Read the model definition and answer for the solid it produces. Units are mm, in the model's axes. A direction names the side the tool comes from. Coordinates: 2 decimals unless noted, no trailing zeros. Order: outer loops, then holes, each group sorted by start corner. A loop starts at its lowest first (then second) coordinate and runs counter-clockwise, first axis right, second up. Notation, with made-up numbers: (3, 2) -> (12, 2) arc R32 ccw to (12, 36) -> close; hole circle Ø11 at (32.25, 29). An arc over 180 degrees is marked (long way). Use CSV: the item, a comma, the result in double quotes.
```python
from build123d import *

# Parameters (mm, degrees)
SKETCH005_R         = 2
EXTRUDE002_DEPTH    = 20
SKETCH002_R         = 7.75
EXTRUDE_DEPTH       = 16
BOX_W               = 8
BOX_H               = 74
BOX_DEPTH           = 120
PAD001_DEPTH        = 20
PAD_DEPTH           = 20
HOLE_D              = 4.4
HOLE_CBORE_D        = 8
HOLE_CBORE_DEPTH    = 2.4
HOLE001_D           = 1.75
HOLE001_CBORE_D     = 3.2
HOLE001_CBORE_DEPTH = 0.96
BOX001_W            = 65
BOX001_H            = 8
BOX001_DEPTH        = 120
BOX002_W            = 2
BOX002_H            = 10
BOX002_DEPTH        = 10
EXTRUDE001_DEPTH    = 8
CHAMFER_SIZE        = 2.5


with BuildPart() as extrude002:
    # Sketch005 (on Face21 of Fusion001) → Extrude002 (new body)
    with BuildSketch(Plane(origin=(-8, 0, 0), x_dir=(0, -1, 0), z_dir=(-1, 0, 0))):
        with Locations((-55, 60)):
            Circle(SKETCH005_R)
        with Locations((-22, 60)):
            Circle(SKETCH005_R)
    extrude(amount=EXTRUDE002_DEPTH)


with BuildPart() as extrude002_1:
    # Extrude002 placement: moved
    add(extrude002.part.moved(Location((16, 0, 0))))


with BuildPart() as extrude_body:
    # Sketch002 (on Face9 of Fusion) → Extrude (new body)
    with BuildSketch(Plane(origin=(0, 74, 0), x_dir=(-1, 0, 0), z_dir=(0, 1, 0))):
        with Locations((35, 60)):
            Circle(SKETCH002_R)
    extrude(amount=EXTRUDE_DEPTH)


with BuildPart() as cube:
    # Box → Box (new body)
    with BuildSketch(Plane(origin=(-8, 0, 0), x_dir=(1, 0, 0), z_dir=(0, 0, 1))):
        with Locations((4, 37)):
            Rectangle(BOX_W, BOX_H)
    extrude(amount=BOX_DEPTH)


with BuildPart() as body001:
    # Sketch001 → Pad001 (new body)
    with BuildSketch(Plane.XY):
        Polygon((-88, 8), (-8, 8), (-8, 36), (-78, 36), (-78, 44), (-8, 44), (-8, 66), (-65, 66), (-65, 74), (0, 74), (0, 0), (-88, 0), align=None)
    extrude(amount=PAD001_DEPTH)


with BuildPart() as body001_1:
    # Body001 placement: moved
    add(body001.part.moved(Location((0, 0, 100))))


with BuildPart() as body:
    # Sketch → Pad (new body)
    with BuildSketch(Plane.XY):
        Polygon((-88, 8), (-8, 8), (-8, 36), (-78, 36), (-78, 44), (-8, 44), (-8, 66), (-65, 66), (-65, 74), (0, 74), (0, 0), (-88, 0), align=None)
    extrude(amount=PAD_DEPTH)

    # Hole (through all)
    with Locations(Plane(origin=(-8, 0, 0), x_dir=(0, -1, 0), z_dir=(-1, 0, 0))):
        with Locations((-55, 60), (-22, 60)):
            CounterBoreHole(HOLE_D / 2, HOLE_CBORE_D / 2, HOLE_CBORE_DEPTH)

    # Hole001 (through all)
    with Locations(Plane(origin=(-8, 0, 0), x_dir=(0, -1, 0), z_dir=(-1, 0, 0))):
        with Locations((-55, 60), (-22, 60)):
            CounterBoreHole(HOLE001_D / 2, HOLE001_CBORE_D / 2, HOLE001_CBORE_DEPTH)


with BuildPart() as fusion:
    # Box001 → Box001 (new body)
    with BuildSketch(Plane(origin=(-65, 66, 0), x_dir=(1, 0, 0), z_dir=(0, 0, 1))):
        with Locations((32.5, 4)):
            Rectangle(BOX001_W, BOX001_H)
    extrude(amount=BOX001_DEPTH)

    # Fusion: union Cube, Body001, Body
    add(cube.part)
    add(body001_1.part)
    add(body.part)


with BuildPart() as cube002:
    # Box002 → Box002 (new body)
    with BuildSketch(Plane(origin=(-84, 64, 55), x_dir=(1, 0, 0), z_dir=(0, 0, 1))):
        with Locations((1, 5)):
            Rectangle(BOX002_W, BOX002_H)
    extrude(amount=BOX002_DEPTH)


with BuildPart() as chamfer_body:
    # Sketch003 (on Face9 of Fusion) → Extrude001 (new body)
    with BuildSketch(Plane(origin=(0, 74, 0), x_dir=(-1, 0, 0), z_dir=(0, 1, 0))):
        Polygon((65, 100), (65, 20), (88, 50), (88, 70), align=None)
    extrude(amount=-EXTRUDE001_DEPTH)

    # Cut: cut Cube002
    add(cube002.part, mode=Mode.SUBTRACT)

    # Fusion001: union Extrude body, Fusion
    add(extrude_body.part)
    add(fusion.part)

    # Cut001: cut Extrude002
    add(extrude002_1.part, mode=Mode.SUBTRACT)

    # Chamfer
    chamfer_edges = [chamfer_body.edges().sort_by_distance(p)[0] for p in [
        (-8, 24, 60),
        (-8, 57, 60),
    ]]
    chamfer(chamfer_edges, length=CHAMFER_SIZE)


solid = chamfer_body.part
```
Item 1: The mould has two halves that part along Y. Classify faces 1 (the flat face through (-34, 0, 19)), 2 (the cylindrical face through (-3, 55, 62)), 3 (the flat face through (-65, 70, 10)): +Y half, -Y half, draft (parallel to the pull), parting line (faces both ways), or undercut.
Return value:
face 1,"-Y half"
face 2,"undercut"
face 3,"draft"
Item 2: Straight lines are drawn through the part: line 1 along Y through (x, z) = (-3.45, 60); line 2 along Y through (x, z) = (-54, 103); line 3 along Z through (x, y) = (-1.2, 22). For each, find the intervals that lie inside material, in ascending order.
Return value:
line 1,"y = 0 to 20, 24 to 53, 57 to 74"
line 2,"y = 0 to 8, 36 to 44, 66 to 74"
line 3,"z = 0 to 58, 62 to 120"
Item 3: Find section D-D, the plane x = -16. Give the vertices of the cut face in (y, z).
Return value:
outline,"(0, 0) -> (8, 0) -> (8, 20) -> (0, 20) -> close; (0, 100) -> (8, 100) -> (8, 120) -> (0, 120) -> close; (36, 0) -> (44, 0) -> (44, 20) -> (36, 20) -> close; (36, 100) -> (44, 100) -> (44, 120) -> (36, 120) -> close; (66, 0) -> (74, 0) -> (74, 120) -> (66, 120) -> close"
Item 4: Each of these flat-tipped pins is pushed along its axis until it touches: P1, Ø4, axis at y = 69.5, z = 113.5, coming from the -X side; P2, Ø8, axis at y = 49.5, z = 61.5, coming from the +X side; P3, Ø9, axis at y = 40, z = 112, coming from the -X side; P4, Ø10, axis at x = -47, z = 8.5, coming from the +Y side. Where does it stop, or does it pass through?
Return value:
P1,"stops at x = -65"
P2,"stops at x = 0"
P3,"stops at x = -78"
P4,"stops at y = 74"
Item 5: Find section C-C, the plane z = 60. Give the vertices of the cut face in (x, y), then the cut area to 3 significant figures.
Return value:
outline,"(-88, 66) -> (-84, 66) -> (-84, 74) -> (-88, 74) -> close; (-82, 66) -> (-8, 66) -> (-8, 59.5) -> (-5.5, 57) -> (0, 57) -> (0, 74) -> (-27.25, 74) -> (-27.25, 90) -> (-42.75, 90) -> (-42.75, 74) -> (-82, 74) -> close; (-8, 0) -> (0, 0) -> (0, 20) -> (-5.5, 20) -> (-8, 17.5) -> close; (-8, 26.5) -> (-5.5, 24) -> (0, 24) -> (0, 53) -> (-5.5, 53) -> (-8, 50.5) -> close"
area,"1,390 mm^2"
Item 6: Find section B-B, the plane y = 55. Give the vertices of the cut face in (x, z), then the cut area to 3 significant figures.
Return value:
outline,"(-8, 0) -> (0, 0) -> (0, 58) -> (-5.5, 58) -> (-8, 55.5) -> close; (-8, 64.5) -> (-5.5, 62) -> (0, 62) -> (0, 120) -> (-8, 120) -> close"
area,"922 mm^2"
Item 7: Find section A-A, the plane x = -35. Give the vertices of the cut face in (y, z), then the cut area to 3 significant figures.
Return value:
outline,"(0, 0) -> (8, 0) -> (8, 20) -> (0, 20) -> close; (0, 100) -> (8, 100) -> (8, 120) -> (0, 120) -> close; (36, 0) -> (44, 0) -> (44, 20) -> (36, 20) -> close; (36, 100) -> (44, 100) -> (44, 120) -> (36, 120) -> close; (66, 0) -> (74, 0) -> (74, 52.25) -> (90, 52.25) -> (90, 67.75) -> (74, 67.75) -> (74, 120) -> (66, 120) -> close"
area,"1,850 mm^2"
Item 8: A tool of negligible diameter and unlimited length cuts with its end or side. For faces 4 (the cylindrical face through (-33.32, 81.888, 52.434)), 5 (the flat face through (-47, 4, 20)), 6 (the flat face through (-88, 70, 60)), 7 (the flat face through (-82, 70, 60)), 8 (the flat face through (-49, 8, 10)), from which of +Z, -Z, +X, -X, +Y, -Y can it reach the whole face along a straight path? Write none if from no direction.
Return value:
face 4,"+Y"
face 5,"-X, -Y"
face 6,"+Z, -Z, -X, +Y, -Y"
face 7,"+Y, -Y"
face 8,"+Z, -Z, -X"
